```python
from build123d import *

# Parameters (mm, degrees)
F2_R     = 2.5
F3_DEPTH = 2
F5_DEPTH = 40
F6_R     = 5


with BuildPart() as f3:
    # F2 (on Top) → F3 (new body)
    with BuildSketch(Plane.XY):
        with BuildLine():
            ThreePointArc((5.65, 0), (0, -5.65), (-5.65, 0))
            Line((-5.65, 0), (-30.3692883162, 0))
            Line((-30.3692883162, 0), (-5.65, -26))
            ThreePointArc((-5.65, -26), (0, -31.65), (5.65, -26))
            Line((5.65, -26), (30.3692883162, 0))
            Line((30.3692883162, 0), (5.65, 0))
        make_face()
        with Locations((0, -26)):
            Circle(F2_R, mode=Mode.SUBTRACT)
        with Locations((0, -16)):
            Circle(F2_R, mode=Mode.SUBTRACT)
    extrude(amount=F3_DEPTH)

    # F4 (on face) → F5 (join)
    with BuildSketch(Plane.XY.offset(2)):
        with BuildLine():
            ThreePointArc((5.65, 0), (0, -5.65), (-5.65, 0))
            Line((-5.65, 0), (-7.65, 0))
            ThreePointArc((-7.65, 0), (0, -7.65), (7.65, 0))
            Line((7.65, 0), (5.65, 0))
        make_face()
    extrude(amount=F5_DEPTH)

    # F6
    f6_edges = [f3.edges().sort_by_distance(p)[0] for p in [
        (0, -7.65, 2),
        (-30.369288, 0, 1),
        (-5.65, -26, 1),
        (5.65, -26, 1),
        (30.369288, 0, 1),
    ]]
    fillet(f6_edges, radius=F6_R)

    # F7 (on face) → F8 (revolve, cut)
    with BuildSketch(Plane(origin=(0, 0, 0), x_dir=(-1, 0, 0), z_dir=(0, 1, 0))):
        with BuildLine():
            ThreePointArc((8.65, 14.8333333333), (7.15, 13.3333333333), (8.65, 11.8333333333))
            Line((8.65, 11.8333333333), (8.65, 14.8333333333))
        make_face()
        with BuildLine():
            ThreePointArc((8.65, 30.1666666667), (7.15, 28.6666666667), (8.65, 27.1666666667))
            Line((8.65, 27.1666666667), (8.65, 30.1666666667))
        make_face()
        Polygon((5.65, 41), (6.65, 42), (5.65, 42), align=None)
    revolve(axis=Axis((0, 0, 10.5), (0, 0, -1)), mode=Mode.SUBTRACT)


solid = f3.part
```
The model under review builds one solid part; all positions refer to its coordinate system, in mm. A direction names the side the tool comes from. Round coordinates to 2 decimals unless told otherwise and drop trailing zeros. Loops run counter-clockwise (first coordinate to the right, second up) from the corner with the lowest first, then second, coordinate; pieces in that order, holes last. Notation, with made-up numbers: (10.5, 9) -> (36.5, 9) arc R5 cw to (36.5, 16) -> close; hole circle Ø5 at (-21, -23.75). An arc over 180 degrees is marked (long way). Answer in a Markdown table with one row per item.
1) Consider section D-D, the plane y = -16. Write out the cut boundary in (x, z), plus the area to 3 significant figures.
Taken from the geometry:
| item | result |
|---|---|
| outline | (-15.16, 0) -> (-2.5, 0) -> (-2.5, 2) -> (-15.16, 2) -> close; (2.5, 0) -> (15.16, 0) -> (15.16, 2) -> (2.5, 2) -> close |
| area | 50.6 mm² |
2) Consider section B-B, the plane y = -26. Write out the cut boundary in (x, z).
Taken from the geometry:
| item | result |
|---|---|
| outline | (-5.94, 0) -> (-2.5, 0) -> (-2.5, 2) -> (-5.94, 2) -> close; (2.5, 0) -> (5.94, 0) -> (5.94, 2) -> (2.5, 2) -> close |
3) Consider section A-A, the plane x = 0. Write out the cut boundary in (y, z), plus the area to 3 significant figures.
Taken from the geometry:
| item | result |
|---|---|
| outline | (-31.65, 0) -> (-28.5, 0) -> (-28.5, 2) -> (-31.65, 2) -> close; (-23.5, 0) -> (-18.5, 0) -> (-18.5, 2) -> (-23.5, 2) -> close; (-13.5, 0) -> (-5.65, 0) -> (-5.65, 41) -> (-6.65, 42) -> (-7.65, 42) -> (-7.65, 29.78) arc R1.5 cw to (-7.65, 27.55) -> (-7.65, 14.45) arc R1.5 cw to (-7.65, 12.22) -> (-7.65, 7) arc R5 cw to (-12.65, 2) -> (-13.5, 2) -> close |
| area | 115 mm² |
4) Wall thickness on line 1 along Y through (x, z) = (0, 0.75); line 2 along Z through (x, y) = (15.5, -15.5); line 3 along X through (y, z) = (-3.5, 6.5): over which ranges is each line inside the solid? List them lowest first.
Taken from the geometry:
| item | result |
|---|---|
| line 1 | y = -31.65 to -28.5, -23.5 to -18.5, -13.5 to -5.65 |
| line 2 | z = 0 to 2 |
| line 3 | x = -6.83 to -4.44, 4.44 to 6.83 |
5) Tool access review of faces 1 (the flat face through (5, -12, 2)), 2 (the cylindrical face through (-0.33, -23.52, 0.99)): name each direction out of +Z, -Z, +X, -X, +Y, -Y from which nothing blocks a thin tool from reaching the whole face with its end or side.
Taken from the geometry:
| item | result |
|---|---|
| face 1 | +Z, -Y |
| face 2 | +Z, -Z |
6) Draft analysis for pull direction X (two halves, no side actions). For faces 3 (the cylindrical face through (-0.54, -18.44, 0.99)), 4 (the cylindrical face through (-0.17, -7.65, 35.81)), 5 (the cylindrical face through (23.34, -3.1, 1.01)), state which applies: pulls with the +X half, pulls with the -X half, needs draft (parallel to the pull), parting line crosses it, or undercut.
Taken from the geometry:
| item | result |
|---|---|
| face 3 | undercut |
| face 4 | parting line crosses it |
| face 5 | pulls with the +X half |
7) For pin 1 Ø6 at (y, z) = (-10, 14.5) entering from +X; pin 2 Ø6 at (y, z) = (-5, 27) entering from -X; pin 3 Ø4 at (x, y) = (-12, -15.5) entering from +Z, all flat-tipped, find the tip position at first contact; note any pin that passes through.
Taken from the geometry:
| item | result |
|---|---|
| pin 1 | stops at x = 3.09 |
| pin 2 | stops at x = -7.38 |
| pin 3 | stops at z = 2 |
8) Consider section C-C, the plane z = 15.5. Write out the cut boundary in (x, y).
Taken from the geometry:
| item | result |
|---|---|
| outline | (-7.65, 0) arc R7.65 ccw to (7.65, 0) -> (5.65, 0) arc R5.65 cw to (-5.65, 0) -> close |
